Work out the finished part from the listing and answer in its coordinate system (mm). A direction names the side the tool comes from. Round coordinates to 2 decimals unless told otherwise and drop trailing zeros. Loops run counter-clockwise (first coordinate to the right, second up) from the corner with the lowest first, then second, coordinate; pieces in that order, holes last.
```python
from build123d import *

# Parameters (mm, degrees)
ESQUISSE4_W             = 86
ESQUISSE4_H             = 66
BOSS_EXTRU_3_DEPTH      = 5
ESQUISSE5_W             = 86
ESQUISSE5_H             = 66
ESQUISSE5_W_2           = 80
ESQUISSE5_H_2           = 60
BOSS_EXTRU_5_DEPTH      = 15
ESQUISSE7_W             = 6.326895014
ESQUISSE7_H             = 16.739909725
ENL_V_MAT_EXTRU_3_DEPTH = 15
ESQUISSE8_W             = 7.644998142
ESQUISSE8_H             = 15.55361691
ESQUISSE8_H_2           = 16.608099413
ENL_V_MAT_EXTRU_4_DEPTH = 15


with BuildPart() as part:
    # Esquisse4 → Boss.-Extru.3 (new body)
    with BuildSketch(Plane.XY):
        with Locations((7.16988417, -5.664092664)):
            Rectangle(ESQUISSE4_W, ESQUISSE4_H)
    extrude(amount=BOSS_EXTRU_3_DEPTH)

    # Esquisse5 → Boss.-Extru.5 (add)
    with BuildSketch(Plane.XY.offset(5)):
        with Locations((7.16988417, -5.664092664)):
            Rectangle(ESQUISSE5_W, ESQUISSE5_H)
        with Locations((7.16988417, -5.664092664)):
            Rectangle(ESQUISSE5_W_2, ESQUISSE5_H_2, mode=Mode.SUBTRACT)
    extrude(amount=BOSS_EXTRU_5_DEPTH)

    # Esquisse7 → Enlèv. mat.-Extru.3 (cut)
    with BuildSketch(Plane.ZY.offset(35.83011583)):
        with Locations((14.481550635, -24.644777708)):
            Rectangle(ESQUISSE7_W, ESQUISSE7_H)
    extrude(amount=-ENL_V_MAT_EXTRU_3_DEPTH, mode=Mode.SUBTRACT)

    # Esquisse8 → Enlèv. mat.-Extru.4 (cut)
    with BuildSketch(Plane(origin=(50.16988417, 0, 0), x_dir=(0, 0, -1), z_dir=(1, 0, 0))):
        with Locations((-12.768016569, -25.237924115)):
            Rectangle(ESQUISSE8_W, ESQUISSE8_H)
        with Locations((-12.768016569, -0.457585309)):
            Rectangle(ESQUISSE8_W, ESQUISSE8_H_2)
    extrude(amount=-ENL_V_MAT_EXTRU_4_DEPTH, mode=Mode.SUBTRACT)


solid = part.part
```
1. Find section D-D (y = -23). Write down the section's boundary in (x, z) (3 decimals).
Answer key:
outline: (-35.83, 0) - (50.17, 0) - (50.17, 8.946) - (47.17, 8.946) - (47.17, 5) - (-32.83, 5) - (-32.83, 11.318) - (-35.83, 11.318) - close; (-35.83, 17.645) - (-32.83, 17.645) - (-32.83, 20) - (-35.83, 20) - close; (47.17, 16.591) - (50.17, 16.591) - (50.17, 20) - (47.17, 20) - close
2. Which of the six approach directions +Z, -Z, +X, -X, +Y, -Y give full straight-line access (tool end or side, diameter ignored) to faces 1 (the face through (-34, -16.275, 14)), 2 (the face through (49, 7.846, 13)), 3 (the face through (7, -5, 0)), 4 (the face through (7, 24.336, 12))?
Answer key:
face 1: -X
face 2: +X
face 3: -Z, +X, -X, +Y, -Y
face 4: +Z
3. Find section C-C (y = 18.5). Write down the section's boundary in (x, z), then the cut area to 3 significant figures.
Answer key:
outline: (-35.83, 0) - (50.17, 0) - (50.17, 20) - (47.17, 20) - (47.17, 5) - (-32.83, 5) - (-32.83, 20) - (-35.83, 20) - close
area: 520 mm2
4. Determine the mould class of faces 5 (the face through (50.17, -6, 8)), 6 (the face through (-34, -33.015, 14)), 7 (the face through (7, -35.664, 12)) for opening direction X: +X half, -X half, draft (parallel to the pull), parting line (faces both ways), or undercut.
Answer key:
face 5: +X half
face 6: draft
face 7: undercut
5. Find section B-B (y = 0.5). Write down the section's boundary in (x, z), then the cut area to 3 significant figures.
Answer key:
outline: (-35.83, 0) - (50.17, 0) - (50.17, 8.95) - (47.17, 8.95) - (47.17, 5) - (-32.83, 5) - (-32.83, 20) - (-35.83, 20) - close; (47.17, 16.59) - (50.17, 16.59) - (50.17, 20) - (47.17, 20) - close
area: 497 mm2
6. Consider probe 1 along X at (y, z) = (-28.5, 7.75); probe 2 along Y at (x, z) = (46, 12.5); probe 3 along Z at (x, y) = (-4, -16.5). Determine where each line is inside the solid, lowest interval first.
Answer key:
probe 1: x = -35.83 to -32.83, 47.17 to 50.17
probe 2: y = -38.66 to -35.66, 24.34 to 27.34
probe 3: z = 0 to 5
7. Given pin 1 (6 mm diameter, centred on x = -22, y = 7, fed in from +Z), flat-ended and moving along its own axis, determine where the tip first touches the part or whether it passes through.
Answer key:
pin 1: stops at z = 5
8. Find section A-A (z = 7.5). Write down the section's boundary in (x, y), then the cut area to 3 significant figures.
Answer key:
outline: (-35.83, -38.66) - (50.17, -38.66) - (50.17, 27.34) - (-35.83, 27.34) - close; hole (-32.83, -35.66) - (47.17, -35.66) - (47.17, 24.34) - (-32.83, 24.34) - close
area: 876 mm2
